Part model, mm, in its own coordinate system. A direction names the side the tool comes from. Give positions to 0.01 mm unless a question says otherwise; leave off trailing zeros. Loops run counter-clockwise (first coordinate to the right, second up) from the corner with the lowest first, then second, coordinate; pieces in that order, holes last. Notation, with made-up numbers: (49.5, -28) -> (95.5, -28) arc R24 cw to (95.5, -17) -> close; hole circle Ø3 at (46.25, 0.25). An arc over 180 degrees is marked (long way). Write item = value, one per line.
Autodesk Inventor part; units mm, degrees
ref_plane "YZ Plane" through (0, 0, 0) normal (1, 0, 0) x (0, 1, 0)
ref_plane "XZ Plane" through (0, 0, 0) normal (0, 1, 0) x (-1, 0, 0)
ref_plane "XY Plane" through (0, 0, 0) normal (0, 0, 1) x (1, 0, 0)
sketch "Skizze1" plane through (0, 0, 0) normal (0, 1, 0) x (-1, 0, 0)
  circle A0 centre (0, 0) radius 24
  dimension "d0" = 48
extrude "Extrusion1" add sketch "Skizze1" along normal blind 6.5
sketch "Skizze2" plane through (0, 6.5, 0) normal (0, 1, 0) x (1, 0, 0)
  circle A0 centre (0, 0) radius 24
  line L0 (-20.4878, -12.5) -> (20.4878, -12.5)
  circle A1 centre (0, 0) radius 24
  line L1 (-20.4878, 12.5) -> (20.4878, 12.5)
  line L2 (-24, 0) -> (24, 0) construction
  dimension "d3" = 12.5
  dimension "d4" = 12.5
extrude "Extrusion2" cut sketch "Skizze2" against normal up to surface (6.5 mm away) contours L1 A0 | A0 L0
sketch "Skizze3" plane through (0, 0, 0) normal (0, -1, 0) x (1, 0, 0)
  circle A0 centre (0, 0) radius 11.5
  dimension "d7" = 23
extrude "Extrusion3" add sketch "Skizze3" along normal blind 40.5
sketch "Skizze4" plane through (0, 6.5, 0) normal (0, 1, 0) x (1, 0, 0)
  point P0 (0, 0)
  point P1 (0, 0)
hole "Bohrung1" at (0, 6.5, 0) direction (0, -1, 0) diameter 19 depth 47
sketch "Skizze5" plane through (0, 6.5, 0) normal (0, 1, 0) x (1, 0, 0)
  line L0 (-20.4878, -12.5) -> (20.4878, -12.5)
  point P0 (0, 0)
  point P1 (17.5, 0)
  point P2 (-17.5, 0)
  dimension "d25" = 12.5
  dimension "d26" = 12.5
  dimension "d27" = 17.5
  dimension "d28" = 17.5
hole "Bohrung2" at (17.5, 6.5, 0) at (-17.5, 6.5, 0) direction (0, -1, 0) diameter 5 depth 6.5
fillet "Rundung1" radius 1 1 edges at (-11.5, 0, 0)
chamfer "Fasen1" distance 1 angle 45 1 edges at (-11.5, -40.5, 0)
chamfer "Fasen2" distance 0.5 angle 45 4 edges at (0, 0, -12.5) (-24, 0, 0) (24, 0, 0) (0, 0, 12.5)
properties part number "11" material "Acetalharz, Weiß"
1) Slice it at A-A, the plane z = 0. List the corners of the cut face in (x, y).
Resolved:
outline = (-24, 0.5) -> (-23.5, 0) -> (-20, 0) -> (-20, 6.5) -> (-24, 6.5) -> close; (-15, 0) -> (-12.5, 0) arc R1 cw to (-11.5, -1) -> (-11.5, -39.5) -> (-10.5, -40.5) -> (-9.5, -40.5) -> (-9.5, 6.5) -> (-15, 6.5) -> close; (9.5, -40.5) -> (10.5, -40.5) -> (11.5, -39.5) -> (11.5, -1) arc R1 cw to (12.5, 0) -> (15, 0) -> (15, 6.5) -> (9.5, 6.5) -> close; (20, 0) -> (23.5, 0) -> (24, 0.5) -> (24, 6.5) -> (20, 6.5) -> close
2) Slice it at B-B, the plane x = 17.5. List the corners of the cut face in (y, z).
Resolved:
outline = (0, -12) -> (0.5, -12.5) -> (6.5, -12.5) -> (6.5, -2.5) -> (0, -2.5) -> close; (0, 2.5) -> (6.5, 2.5) -> (6.5, 12.5) -> (0.5, 12.5) -> (0, 12) -> close
3) Drill centre lines: line 1 along X through (y, z) = (4.75, 0); line 2 along X through (y, z) = (-37.5, -0.25). Where is each one in solid material? Low to high. Write a range as [from, to].
Resolved:
line_1 = [-24, -20], [-15, -9.5], [9.5, 15], [20, 24]
line_2 = [-11.5, -9.5], [9.5, 11.5]
4) Drop flat-ended pins along their axis: P1, Ø6, axis at y = -22.5, z = -8, coming from the -X side; P2, Ø4, axis at x = 8.5, y = -20.5, coming from the -Z side; P3, Ø1, axis at x = -4.5, y = -23.5, coming from the +Z side; P4, Ø10, axis at x = 10, z = -5.5, coming from the -Y side. Give the stop position or say it passes through.
Resolved:
P1 = -10.36
P2 = -9.49
P3 = 10.78
P4 = -40.5
5) Slice it at C-C, the plane y = 3.5. List the corners of the cut face in (x, z).
Resolved:
outline = (-20.49, -12.5) -> (20.49, -12.5) arc R24 ccw to (20.49, 12.5) -> (-20.49, 12.5) arc R24 ccw to start; hole circle Ø5 at (-17.5, 0); hole circle Ø19 at (0, 0); hole circle Ø5 at (17.5, 0)
6) Pull direction Z, two halves, no side cores. Call faces 1 (the face through (23.64, 0.14, 0.18)), 2 (the face through (8.43, -17.33, 4.38)), 3 (the face through (-5, 6.5, 9)): pulls with the +Z half, pulls with the -Z half, needs draft (parallel to the pull), parting line crosses it, or undercut.
Resolved:
face_1 = parting line crosses it
face_2 = undercut
face_3 = needs draft
7) Slice it at D-D, the plane y = -17. List the corners of the cut face in (x, z), and give its area (3 significant figures).
Resolved:
outline = circle Ø23 at (0, 0); hole circle Ø19 at (0, 0)
area = 132 mm²
8) Which spindle directions (+Z, -Z, +X, -X, +Y, -Y) get a long thin tool onto all of the face, cutting with end or side? Do faces 4 (the face through (24, 3, 0)), 5 (the face through (-1.5, -20, -11.4)). Say none if no direction does.
Resolved:
face_4 = +X, +Y, -Y
face_5 = -Y
